Could you check a few things on this model? Use its own coordinates, in mm. Face numbers are marked on the shaded views. A direction names the side the tool comes from. Give positions to 0.01 mm unless a question says otherwise; leave off trailing zeros. Write each loop counter-clockwise with the first axis right and the second up, starting at its lowest first coordinate (ties: lowest second). Pieces come first, ordered by that corner, then holes. Notation, with made-up numbers: (45.5, 31) - (69.5, 31) arc R27 cw to (69.5, 55) - close; hole circle Ø8 at (11.5, 15). An arc over 180 degrees is marked (long way). Write item = value, one per line.
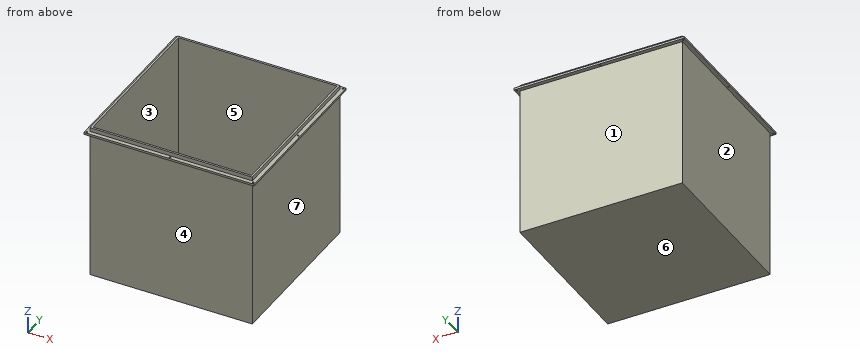
from build123d import *

# Parameters (mm, degrees)
F0_W     = 820
F0_H     = 820
F1_DEPTH = 790
F2_T     = -10
F4_W     = 860
F4_H     = 860
F4_W_2   = 820
F4_H_2   = 820
F5_DEPTH = 10
F7_D     = 8


with BuildPart() as f1:
    # F0 (on Top) → F1 (new body)
    with BuildSketch(Plane.XY):
        Rectangle(F0_W, F0_H)
    extrude(amount=F1_DEPTH)

    # F2
    f2_openings = [f1.faces().sort_by_distance(p)[0] for p in [
        (0, 0, 790),
    ]]
    offset(amount=F2_T, openings=f2_openings)

    # F4 (on offset) → F5 (join)
    with BuildSketch(Plane.XY.offset(770)):
        Rectangle(F4_W, F4_H)
        Rectangle(F4_W_2, F4_H_2, mode=Mode.SUBTRACT)
    extrude(amount=-F5_DEPTH)

    # F7 (through all)
    with Locations(Plane.XY.offset(770)):
        with Locations((0, 420), (-420, 420), (-420, 0), (-420, -420), (0, -420), (420, 0), (420, -420), (420, 420)):
            Hole(F7_D / 2)


solid = f1.part
1. For pin 1 (12 mm diameter, centred on y = -330.5, z = 414.5, fed in from -X); pin 2 (6 mm diameter, centred on x = 245.5, y = -316, fed in from +Z); pin 3 (2 mm diameter, centred on y = 200, z = 331.5, fed in from +X); pin 4 (4 mm diameter, centred on x = 20.5, y = -284.5, fed in from -Z), each with a flat end and sliding along its axis, tell me the tip position at first contact or that it passes through.
Filled sheet:
pin_1 = -410
pin_2 = 10
pin_3 = 410
pin_4 = 0
2. Which directions (+Z, -Z, +X, -X, +Y, -Y) give clear straight access to the entire face, cutting with the end or side of a thin tool? Please do the marked faces 4, 5, 6 and 7.
Filled sheet:
face_4 = -Z, +X, -X, -Y
face_5 = +Z
face_6 = -Z, +X, -X, +Y, -Y
face_7 = -Z, +X, +Y, -Y
3. Thinking about a two-plate mould opening in Y: for the marked faces 1, 2 and 3, which applies, pulls with the +Y half, pulls with the -Y half, needs draft (parallel to the pull), parting line crosses it, or undercut?
Filled sheet:
face_1 = pulls with the +Y half
face_2 = needs draft
face_3 = undercut
4. If we section it at A-A, the plane z = 250: Please give me the cut outline in (x, y), and give its area (3 significant figures).
Filled sheet:
outline = (-410, -410) - (410, -410) - (410, 410) - (-410, 410) - close; hole (-400, -400) - (400, -400) - (400, 400) - (-400, 400) - close
area = 32,400 mm2
5. If we section it at B-B, the plane x = 137.5: Please give me the cut outline in (y, z), and give its area (3 significant figures).
Filled sheet:
outline = (-430, 760) - (-410, 760) - (-410, 0) - (410, 0) - (410, 760) - (430, 760) - (430, 770) - (410, 770) - (410, 790) - (400, 790) - (400, 10) - (-400, 10) - (-400, 790) - (-410, 790) - (-410, 770) - (-430, 770) - close
area = 24,200 mm2
6. I need wall thicknesses on line 1 (X direction, y = -420, z = 765); line 2 (Y direction, x = 184, z = 485.5). Which ranges of each line are inside material? Lowest first, please.
Filled sheet:
line_1 = -430 to -424, -416 to -4, 4 to 416, 424 to 430
line_2 = -410 to -400, 400 to 410
